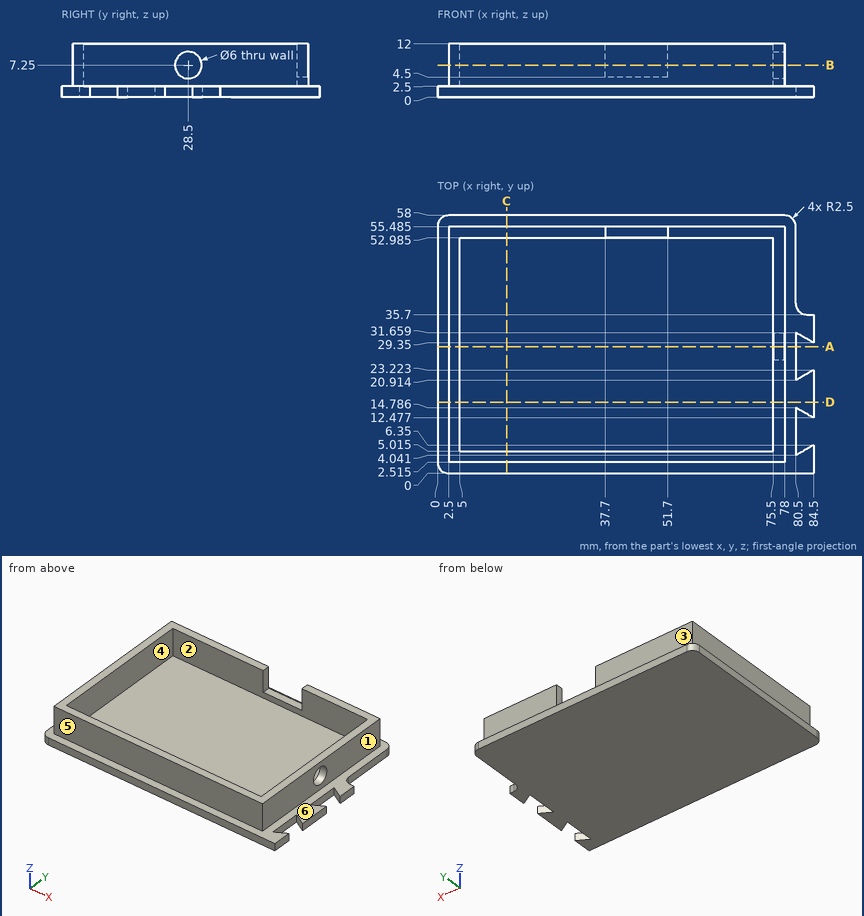
Could you check a few things on this drawing? It's one solid part, dimensions in mm from its lowest x, y, z. A direction names the side the tool comes from. Coordinates: 2 decimals unless noted, no trailing zeros. Write each loop counter-clockwise with the first axis right and the second up, starting at its lowest first coordinate (ties: lowest second). Pieces come first, ordered by that corner, then holes. Notation, with made-up numbers: (66.5, -22.75) - (94.5, -22.75) arc R16 cw to (94.5, -6.75) - close; hole circle Ø10 at (34, -25.75). An arc over 180 degrees is marked (long way). Return JSON: item names as keys, results as strings. Group by question number.
Item 1: If we section it at D-D (y = 16): Write out the boundary of the cut face in (x, z), then the cut area to 3 significant figures.
Item 2: Please list where these lines run through material, in increasing order: probe 1 along Y at (x, z) = (21, 7.75) (1 decimal); probe 2 along X at (y, z) = (24.5, 7.75); probe 3 along Z at (x, y) = (76.9, 28.5).
Item 3: I'm going to push flat-ended pins straight in: pin 1 Ø1.2 at (y, z) = (46.5, 1) entering from +X; pin 2 Ø5.5 at (y, z) = (28.5, 7.25) entering from -X; pin 3 Ø5 at (x, z) = (46.5, 6) entering from +Y (3 decimals). Where does each tip first touch, or does it pass through?
Item 4: If we section it at B-B (z = 7.25): Write out the boundary of the cut face in (x, y) (1 decimal).
Item 5: If we section it at C-C (x = 15.5): Write out the boundary of the cut face in (y, z) (1 decimal).
Item 6: If we section it at A-A (y = 28.5): Write out the boundary of the cut face in (x, z).
Item 7: Which directions (+Z, -Z, +X, -X, +Y, -Y) give clear straight access to the entire face, cutting with the end or side of a thin tool? Please do the marked faces 1, 2 and 3.
Item 8: We'd pull the mould along Y, two halves only. Please class the marked faces 4, 5 and 6: pulls with the +Y half, pulls with the -Y half, needs draft (parallel to the pull), parting line crosses it, or undercut.
Return value:
{
 "1": {"outline": "(0, 0) - (84.5, 0) - (84.5, 2.5) - (78, 2.5) - (78, 12) - (75.5, 12) - (75.5, 2.5) - (5, 2.5) - (5, 12) - (2.5, 12) - (2.5, 2.5) - (0, 2.5) - close", "area": "259 mm^2"},
 "2": {"probe 1": "y = 2.5 to 5, 53 to 55.5", "probe 2": "x = 2.5 to 5, 75.5 to 78", "probe 3": "z = 0 to 4.25, 10.25 to 12"},
 "3": {"pin 1": "stops at x = 80.5", "pin 2": "stops at x = 2.5", "pin 3": "stops at y = 55.485"},
 "4": {"outline": "(2.5, 2.5) - (78, 2.5) - (78, 25.5) - (75.5, 25.5) - (75.5, 5) - (5, 5) - (5, 53) - (37.7, 53) - (37.7, 55.5) - (2.5, 55.5) - close; (51.7, 53) - (75.5, 53) - (75.5, 31.5) - (78, 31.5) - (78, 55.5) - (51.7, 55.5) - close"},
 "5": {"outline": "(0, 0) - (58, 0) - (58, 2.5) - (55.5, 2.5) - (55.5, 12) - (53, 12) - (53, 2.5) - (5, 2.5) - (5, 12) - (2.5, 12) - (2.5, 2.5) - (0, 2.5) - close"},
 "6": {"outline": "(0, 0) - (80.5, 0) - (80.5, 2.5) - (78, 2.5) - (78, 4.25) - (75.5, 4.25) - (75.5, 2.5) - (5, 2.5) - (5, 12) - (2.5, 12) - (2.5, 2.5) - (0, 2.5) - close; (75.5, 10.25) - (78, 10.25) - (78, 12) - (75.5, 12) - close"},
 "7": {"face 1": "+Z, +X, +Y, -Y", "face 2": "+Z", "face 3": "+Z, +X, -X, +Y"},
 "8": {"face 4": "undercut", "face 5": "pulls with the -Y half", "face 6": "needs draft"}
}
